from build123d import *

# Parameters (mm, degrees)
F1_DEPTH = 20
F3_R     = 25
F2_DEPTH = 20.001
F4_R     = 10
F5_DEPTH = 100


with BuildPart() as f1:
    # F0 (on Top) → F1 (new body)
    with BuildSketch(Plane.XY):
        with BuildLine():
            ThreePointArc((12.5, -48.412292), (39.528471, -30.618622), (50, 0))
            ThreePointArc((50, 0), (39.528471, 30.618622), (12.5, 48.412292))
            ThreePointArc((12.5, 48.412292), (-50, 0), (12.5, -48.412292))
        make_face()
        with BuildLine():
            ThreePointArc((12.5, 48.412292), (39.528471, 30.618622), (50, 0))
            Line((50, 0), (75, 0))
            ThreePointArc((75, 0), (84.690689, 19.764235), (106.25, 24.206146))
            Line((106.25, 24.206146), (12.5, 48.412292))
        make_face()
        with BuildLine():
            Line((75, 0), (50, 0))
            ThreePointArc((50, 0), (39.528471, -30.618622), (12.5, -48.412292))
            Line((12.5, -48.412292), (106.25, -24.206146))
            ThreePointArc((106.25, -24.206146), (84.690689, -19.764235), (75, 0))
        make_face()
        with BuildLine():
            ThreePointArc((106.25, 24.206146), (84.690689, 19.764235), (75, 0))
            ThreePointArc((75, 0), (84.690689, -19.764235), (106.25, -24.206146))
            ThreePointArc((106.25, -24.206146), (119.764235, -15.309311), (125, 0))
            ThreePointArc((125, 0), (119.764235, 15.309311), (106.25, 24.206146))
        make_face()
    extrude(amount=F1_DEPTH)

    # F3 (on face) → F2 (cut, through all)
    with BuildSketch(Plane.XY.offset(20)):
        Circle(F3_R)
    extrude(amount=-F2_DEPTH, mode=Mode.SUBTRACT)

    # F4 (on face) → F5 (join)
    with BuildSketch(Plane.XY.offset(20)):
        with Locations((100, 0)):
            Circle(F4_R)
    extrude(amount=F5_DEPTH)


solid = f1.part
Geometry check sheet. Reference: the model listing, model coordinates, mm. A direction names the side the tool comes from. Give positions to 0.01 mm unless a question says otherwise; leave off trailing zeros. Write each loop counter-clockwise with the first axis right and the second up, starting at its lowest first coordinate (ties: lowest second). Pieces come first, ordered by that corner, then holes. Notation, with made-up numbers: M -39.75,-22.5 L -15.75,-22.5 A20 ccw -15.75,6.5 Z; hole C -17,-14 d8. An arc over 180 degrees is marked long. One line per question, with ' | ' between items.
1. Scan lines: line 1 along Y through (x, z) = (0, 10); line 2 along Z through (x, y) = (62, 10); line 3 along Y through (x, z) = (100.5, 36). Record each from-to range of solid material in increasing order. Write a range as from..to.
Ans:
line 1: -50..-25, 25..50 | line 2: 0..20 | line 3: -9.99..9.99
2. Cross-section at C-C (z = 87.5). Enter the section's corners in (x, y).
Ans:
outline: C 100,0 d20
3. Cross-section at A-A (x = 0). Enter the section's corners in (y, z), plus the area to 3 significant figures.
Ans:
outline: M -50,0 L -25,0 L -25,20 L -50,20 Z; M 25,0 L 50,0 L 50,20 L 25,20 Z | area: 1,000 mm2
4. Cross-section at D-D (x = 100). Enter the section's corners in (y, z), plus the area to 3 significant figures.
Ans:
outline: M -25.82,0 L 25.82,0 L 25.82,20 L 10,20 L 10,120 L -10,120 L -10,20 L -25.82,20 Z | area: 3,030 mm2
5. Cross-section at B-B (y = 18). Enter the section's corners in (x, z).
Ans:
outline: M -46.65,0 L -17.35,0 L -17.35,20 L -46.65,20 Z; M 17.35,0 L 117.35,0 L 117.35,20 L 17.35,20 Z
6. Gauge pin test, flat ends, axial feed: pin 1 (1.5 mm diameter, centred on x = 102, z = 49, fed in from +Y); pin 2 (10 mm diameter, centred on x = 37, z = 27.5, fed in from -Y); pin 3 (5 mm diameter, centred on x = 15.5, y = 23, fed in from +Z); pin 4 (1 mm diameter, centred on y = -1.5, z = 105.5, fed in from +X). Record the tip position at first contact, or that the pin passes through.
Ans:
pin 1: y = 9.92 | pin 2: through | pin 3: z = 20 | pin 4: x = 109.95
7. Set-up check for faces 1 (the face through (-49.984, 1.276, 9.86)), 2 (the face through (90, 0, 69)): record each of +Z, -Z, +X, -X, +Y, -Y from which the full face is reachable in a straight line by a thin tool's end or side.
Ans:
face 1: +Z, -Z | face 2: +Z
8. Mould release check, pull along Y, two halves, no side actions. Record for faces 3 (the face through (23.846, 7.509, 10.14)), 4 (the face through (60.03, 36.14, 9.86)), 5 (the face through (100, 0, 120)): released by +Y, released by -Y, zero draft, split by the parting line, or undercut.
Ans:
face 3: undercut | face 4: released by +Y | face 5: zero draft
